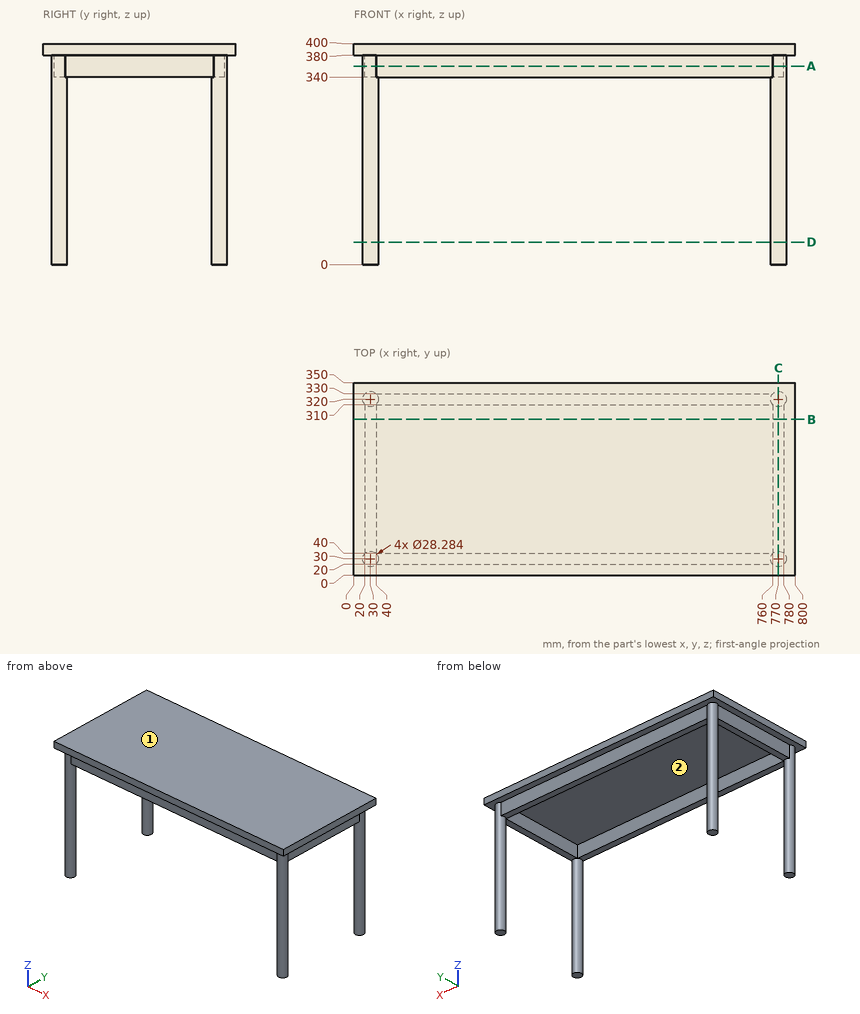
Geometry: see drawing. Coordinates: mm, zero at the bounding-box minimum. Round coordinates to 2 decimals unless told otherwise and drop trailing zeros. Order: outer loops, then holes, each group sorted by start corner. A loop starts at its lowest first (then second) coordinate and runs counter-clockwise, first axis right, second up. Notation, with made-up numbers: (50.25, 16.25) -> (64.25, 16.25) arc R20 cw to (64.25, 33.25) -> close; hole circle Ø7 at (22, 59). An arc over 180 degrees is marked (long way). Answer as CSV lines item,"result".
Item 1: Pull-direction query (X, two-part tool) for the marked faces 1 and 2; classes: pulls with the +X half, pulls with the -X half, needs draft (parallel to the pull), parting line crosses it, or undercut.
A:
face 1,"needs draft"
face 2,"undercut"
Item 2: Section B-B, the plane y = 283. Return loops of the section in (x, z).
A:
outline,"(0, 380) -> (20, 380) -> (20, 340) -> (40, 340) -> (40, 380) -> (760, 380) -> (760, 340) -> (780, 340) -> (780, 380) -> (800, 380) -> (800, 400) -> (0, 400) -> close"
Item 3: Section D-D, the plane z = 40.5. Return loops of the section in (x, y).
A:
outline,"circle Ø28.28 at (30, 30); circle Ø28.28 at (30, 320); circle Ø28.28 at (770, 30); circle Ø28.28 at (770, 320)"
Item 4: Line query: L1, parallel to X at y = 272, z = 353; L2, parallel to Z at x = 305, y = 104.5; L3, parallel to Y at x = 761, z = 59. Output: solid intervals per line, ascending.
A:
L1,"20 to 40, 760 to 780"
L2,"380 to 400"
L3,"19.09 to 40.91, 309.09 to 330.91"
Item 5: Pin query (flat end, axial travel): pin 1 Ø20 at (y, z) = (192, 363) entering from +X; pin 2 Ø12 at (x, z) = (471, 357) entering from -Y; pin 3 Ø12 at (x, z) = (456, 366.5) entering from +Y. Return the tip coordinate at first contact, or that it passes through.
A:
pin 1,"x = 780"
pin 2,"y = 20"
pin 3,"y = 330"
Item 6: Section C-C, the plane x = 770. Return loops of the section in (y, z).
A:
outline,"(0, 380) -> (15.86, 380) -> (15.86, 0) -> (44.14, 0) -> (44.14, 340) -> (305.86, 340) -> (305.86, 0) -> (334.14, 0) -> (334.14, 380) -> (350, 380) -> (350, 400) -> (0, 400) -> close"
Item 7: Section A-A, the plane z = 360. Return loops of the section in (x, y), plus the area to 3 significant figures.
A:
outline,"(20, 40) arc R14.14 ccw to (40, 20) -> (760, 20) arc R14.14 ccw to (780, 40) -> (780, 310) arc R14.14 ccw to (760, 330) -> (40, 330) arc R14.14 ccw to (20, 310) -> close; hole (40, 40) -> (760, 40) -> (760, 310) -> (40, 310) -> close"
area,"41,700 mm²"
